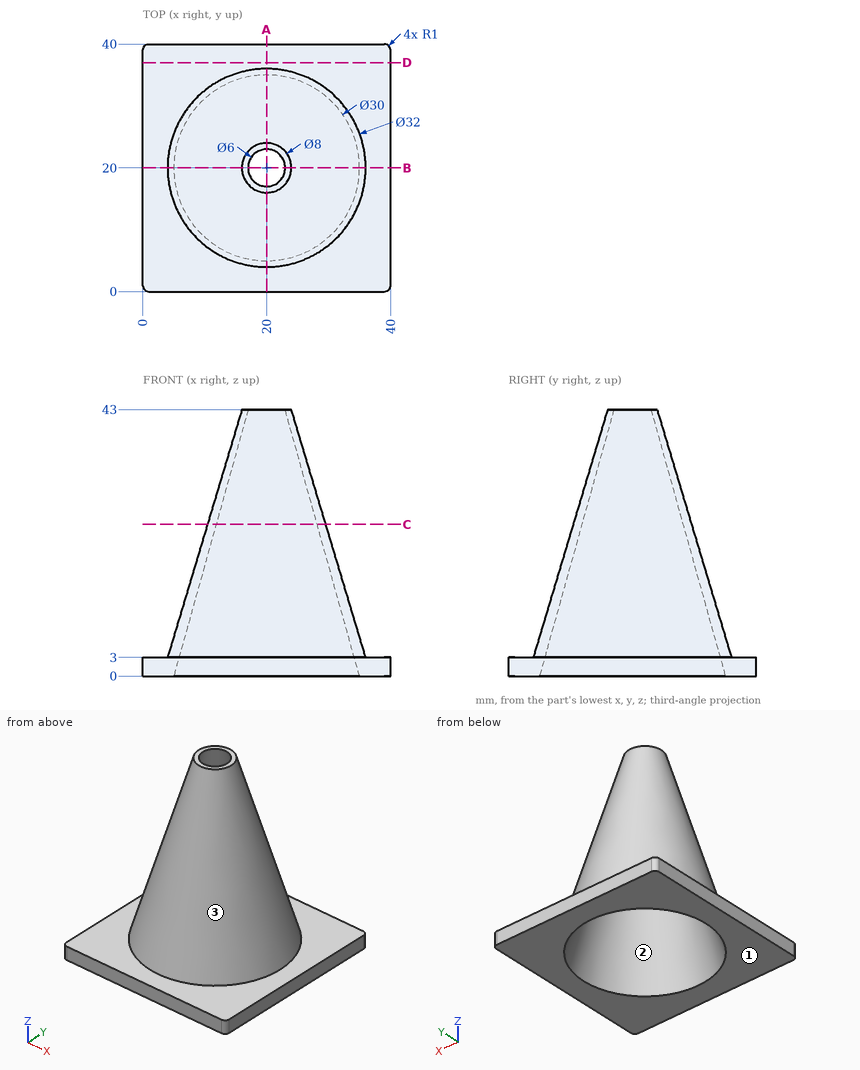
The figure shows three views and two pictorial views of one solid part (mm, origin at its lowest corner). Answer the questions. Give positions to 0.01 mm unless a question says otherwise; leave off trailing zeros. Write each loop counter-clockwise with the first axis right and the second up, starting at its lowest first coordinate (ties: lowest second). Pieces come first, ordered by that corner, then holes. Notation, with made-up numbers: (7.25, -34) - (45.25, -34) arc R30 ccw to (45.25, 1) - close; hole circle Ø10 at (27.25, 17.25). An arc over 180 degrees is marked (long way). Use CSV: the item, a comma, the result in double quotes. Start each with the question number.
Item 1: The mould has two halves that part along Y. Classify the marked faces 1, 2 and 3: pulls with the +Y half, pulls with the -Y half, needs draft (parallel to the pull), parting line crosses it, or undercut.
Item 2: Consider line 1 (Z direction, x = 15.5, y = 35.5); line 2 (X direction, y = 17, z = 38.5); line 3 (X direction, y = 21.5, z = 24.5). Determine where each line is inside the solid, lowest interval first.
Item 3: The part is cut by section C-C, the plane z = 24.5. Give the vertices of the cut face in (x, y), and give its area (3 significant figures).
Item 4: Flat-ended cylindrical pins translate along their axes: P1, Ø2, axis at y = 19, z = 20, coming from the -X side; P2, Ø10, axis at y = 10.5, z = 14.5, coming from the -X side; P3, Ø3, axis at x = 33, z = 8.5, coming from the -Y side. Find the tip coordinate at first contact, or state that the pin passes through.
Item 5: The part is cut by section D-D, the plane y = 37. Give the vertices of the cut face in (x, z).
Item 6: The part is cut by section A-A, the plane x = 20. Give the vertices of the cut face in (y, z).
Taken from the geometry:
1,face 1,"needs draft"
1,face 2,"undercut"
1,face 3,"parting line crosses it"
2,line 1,"0 to 3"
2,line 2,"15.57 to 16.98, 23.02 to 24.43"
2,line 3,"10.57 to 11.98, 28.02 to 29.43"
3,outline,"circle Ø19.1 at (20, 20); hole circle Ø16.33 at (20, 20)"
3,area,"77.2 mm2"
4,P1,"x = 8.83"
4,P2,"x = 7.73"
4,P3,"y = 11.28"
5,outline,"(0, 0) - (40, 0) - (40, 3) - (0, 3) - close"
6,outline,"(0, 0) - (5, 0) - (17, 43) - (16, 43) - (4, 3) - (0, 3) - close; (23, 43) - (35, 0) - (40, 0) - (40, 3) - (36, 3) - (24, 43) - close"
